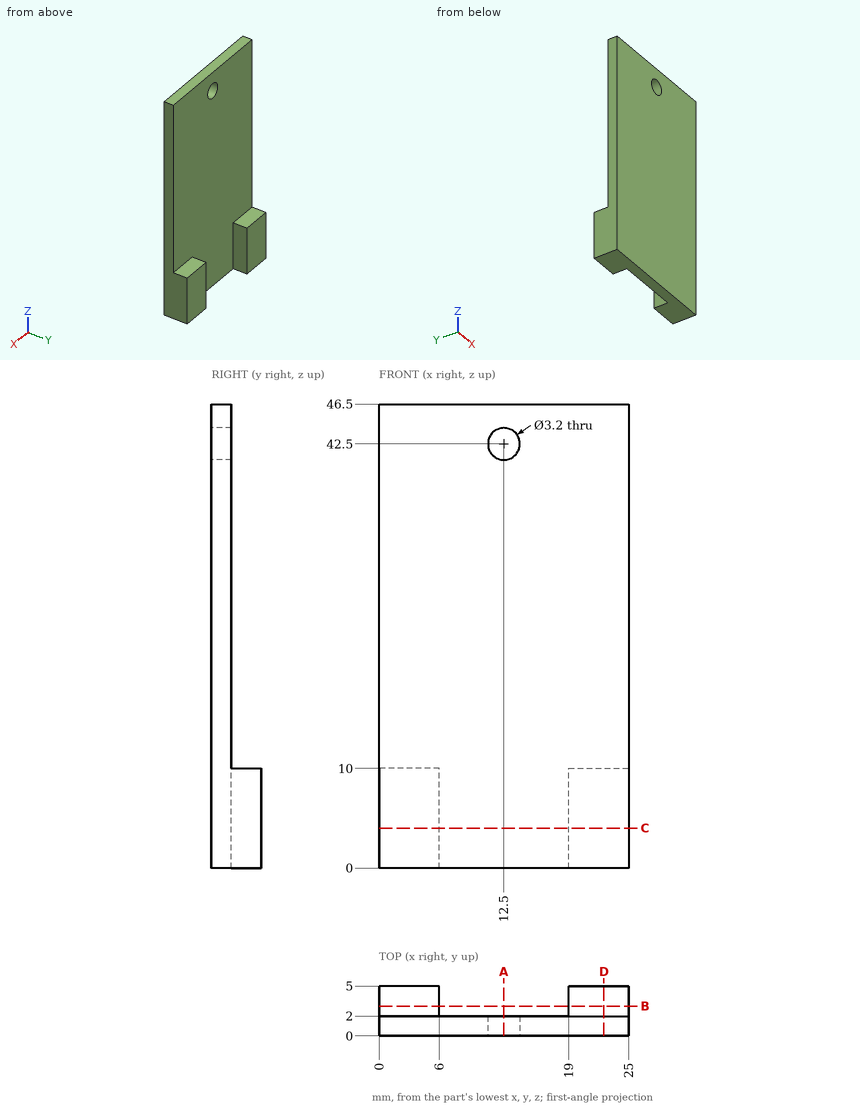
For this review, use the dimensioned drawing (mm, ordinates from the lowest corner) and the shaded views. Give positions to 0.01 mm unless a question says otherwise; leave off trailing zeros. Order: outer loops, then holes, each group sorted by start corner. A loop starts at its lowest first (then second) coordinate and runs counter-clockwise, first axis right, second up. Notation, with made-up numbers: M 22.5,6 L 31.5,6 A23 ccw 31.5,30 Z; hole C 55.25,39 d6. An arc over 180 degrees is marked long. Use one line per item in the form item = value. Start each with the question number.
Item 1: We need section A-A on x = 12.5. Give the boundary of the cut face in (y, z).
Item 2: We need section B-B on y = 3. Give the boundary of the cut face in (x, z), plus the area to 3 significant figures.
Item 3: To check wall thickness, follow line 1 along Z through (x, y) = (12.5, 0.7); line 2 along Y through (x, z) = (9, 37); line 3 along Z through (x, y) = (13.5, 1.5). State the ranges of each line that lie inside material, in increasing order. Write a range as from..to.
Item 4: We need section D-D on x = 22.5. Give the boundary of the cut face in (y, z).
Item 5: Insertion check: pin 1 Ø1.9 at (x, z) = (12.5, 42.5) entering from +Y; pin 2 Ø7.5 at (x, z) = (15.5, 28.5) entering from +Y; pin 3 Ø0.9 at (x, y) = (2.5, 3) entering from +Z. Each pin has a flat end and moves straight along its axis. Give the tip position at first contact, or say it passes through.
Item 6: We need section C-C on z = 4. Give the boundary of the cut face in (x, y), plus the area to 3 significant figures.
Completed:
q1.outline = M 0,0 L 2,0 L 2,40.9 L 0,40.9 Z; M 0,44.1 L 2,44.1 L 2,46.5 L 0,46.5 Z
q2.outline = M 0,0 L 6,0 L 6,10 L 0,10 Z; M 19,0 L 25,0 L 25,10 L 19,10 Z
q2.area = 120 mm²
q3.line_1 = 0..40.9, 44.1..46.5
q3.line_2 = 0..2
q3.line_3 = 0..41.25, 43.75..46.5
q4.outline = M 0,0 L 5,0 L 5,10 L 2,10 L 2,46.5 L 0,46.5 Z
q5.pin_1 = through
q5.pin_2 = 2
q5.pin_3 = 10
q6.outline = M 0,0 L 25,0 L 25,5 L 19,5 L 19,2 L 6,2 L 6,5 L 0,5 Z
q6.area = 86.0 mm²
